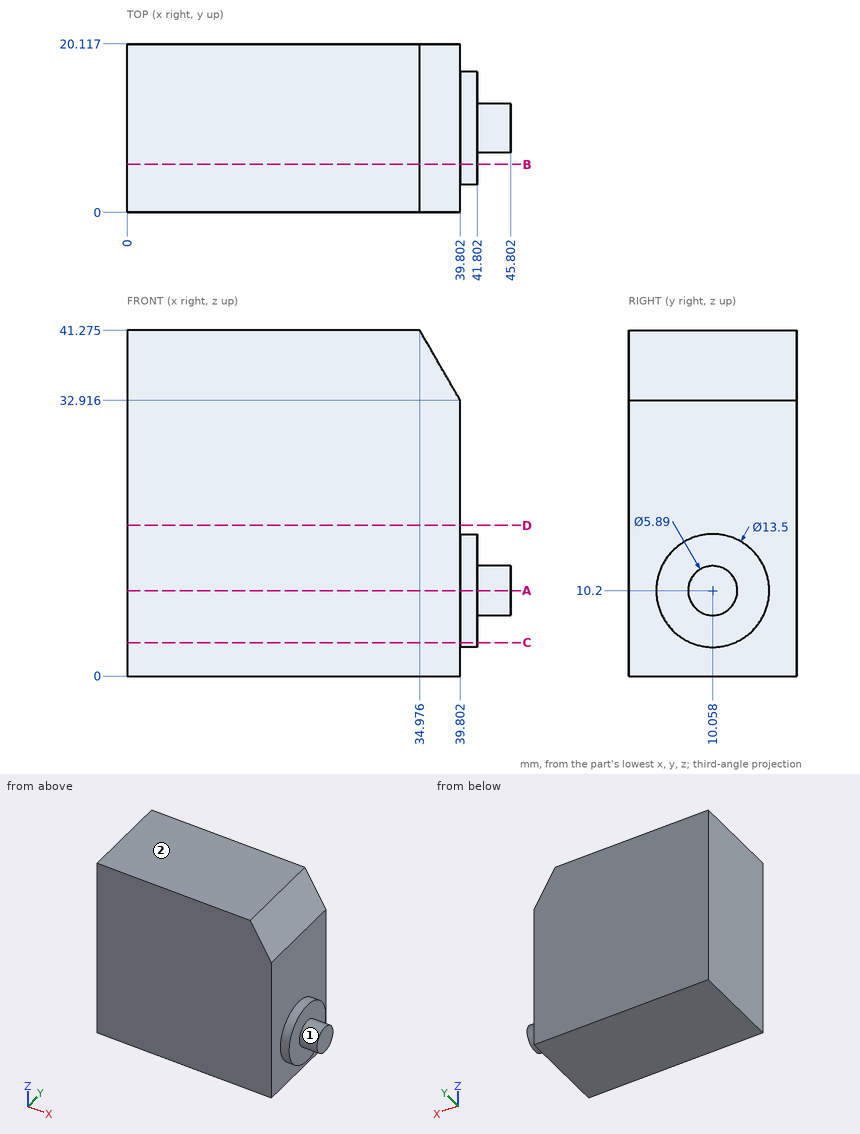
Answer from the drawing. Dimensions are ordinates in mm from the lowest x, y and z of the part. A direction names the side the tool comes from. Round coordinates to 2 decimals unless told otherwise and drop trailing zeros. Loops run counter-clockwise (first coordinate to the right, second up) from the corner with the lowest first, then second, coordinate; pieces in that order, holes last. Notation, with made-up numbers: M 40.5,55 L 73.5,55 A19 ccw 73.5,87 Z; hole C 57.5,-5.75 d4. An arc over 180 degrees is marked long. One line per question, with ' | ' between items. Start each with the question number.
(1) A cutting plane is placed at A-A on z = 10.2. Write down the section's boundary in (x, y).
(2) A tool of negligible diameter and unlimited length cuts with its end or side. For the marked faces 1 and 2, from which of +Z, -Z, +X, -X, +Y, -Y can it reach the whole face along a straight path? Write none if from no direction.
(3) A cutting plane is placed at C-C on z = 4. Write down the section's boundary in (x, y), plus the area to 3 significant figures.
(4) Find the intervals of material crossed by line 1 (X direction, y = 16.5, z = 11); line 2 (X direction, y = 2, z = 23); line 3 (Z direction, x = 38, y = 15.5) (1 decimal), in increasing order.
(5) A cutting plane is placed at D-D on z = 18. Write down the section's boundary in (x, y), plus the area to 3 significant figures.
(6) A cutting plane is placed at B-B on y = 5.75. Write down the section's boundary in (x, z) (1 decimal).
(7) Flat-ended cylindrical pins translate along their axes: pin 1 Ø5 at (y, z) = (11, 29) entering from +X; pin 2 Ø12 at (y, z) = (16, 17.5) entering from +X. Find the tip coordinate at first contact, or state that the pin passes through.
Geometry check:
1) outline: M 0,0 L 39.8,0 L 39.8,3.31 L 41.8,3.31 L 41.8,7.11 L 45.8,7.11 L 45.8,13 L 41.8,13 L 41.8,16.81 L 39.8,16.81 L 39.8,20.12 L 0,20.12 Z
2) face 1: +X | face 2: +Z, +X, -X, +Y, -Y
3) outline: M 0,0 L 39.8,0 L 39.8,7.39 L 41.8,7.39 L 41.8,12.73 L 39.8,12.73 L 39.8,20.12 L 0,20.12 Z | area: 811 mm²
4) line 1: x = 0 to 41.8 | line 2: x = 0 to 39.8 | line 3: z = 0 to 36
5) outline: M 0,0 L 39.8,0 L 39.8,20.12 L 0,20.12 Z | area: 801 mm²
6) outline: M 0,0 L 39.8,0 L 39.8,5 L 41.8,5 L 41.8,15.4 L 39.8,15.4 L 39.8,32.9 L 35,41.3 L 0,41.3 Z
7) pin 1: stops at x = 39.8 | pin 2: stops at x = 41.8
